The listing builds one solid part. Answer for the finished solid, in the listing's coordinates (mm). Face numbers are marked on the shaded views. A direction names the side the tool comes from. Round coordinates to 2 decimals unless told otherwise and drop trailing zeros. Order: outer loops, then holes, each group sorted by start corner. A loop starts at its lowest first (then second) coordinate and runs counter-clockwise, first axis right, second up. Notation, with made-up numbers: M 28.5,65.5 L 34.5,65.5 A22 ccw 34.5,96.5 Z; hole C -35,4 d1. An arc over 180 degrees is marked long. Write item = value, one per line. Start each with the question number.
(1) Straight lines are drawn through the part: probe 1 along Z at (x, y) = (-19.5, 24) (3 decimals); probe 2 along Z at (x, y) = (-16, 68); probe 3 along Z at (x, y) = (73.5, 7). For each, find the intervals that lie inside material, in ascending order. Write a range as from..to.
(2) A cutting plane is placed at A-A, the plane z = 56. Determine the outline of the cut face in (x, y).
(3) A cutting plane is placed at D-D, the plane x = 10. Determine the outline of the cut face in (y, z), and give its area (3 significant figures).
(4) For a pull along Y with two mould halves and no side action, classify the marked faces 6, 7, 8 and 9 as released by +Y, released by -Y, zero draft, split by the parting line, or undercut.
(5) Each of these flat-tipped pins is pushed along its axis until it touches: pin 1 (1.5 mm diameter, centred on x = 67.5, z = 33, fed in from -Y); pin 2 (9 mm diameter, centred on x = -15, y = 4, fed in from +Z); pin 3 (4 mm diameter, centred on y = 12.5, z = 11.5, fed in from +X); pin 4 (5 mm diameter, centred on y = 40, z = 80, fed in from +X). Where does it stop, or does it pass through?
(6) Which of the six approach directions +Z, -Z, +X, -X, +Y, -Y give full straight-line access (tool end or side, diameter ignored) to the marked faces 1, 2, 3, 4 and 5?
(7) A cutting plane is placed at B-B, the plane y = 20. Determine the outline of the cut face in (x, z) (3 decimals).
(8) A cutting plane is placed at C-C, the plane z = 83.5. Determine the outline of the cut face in (x, y).
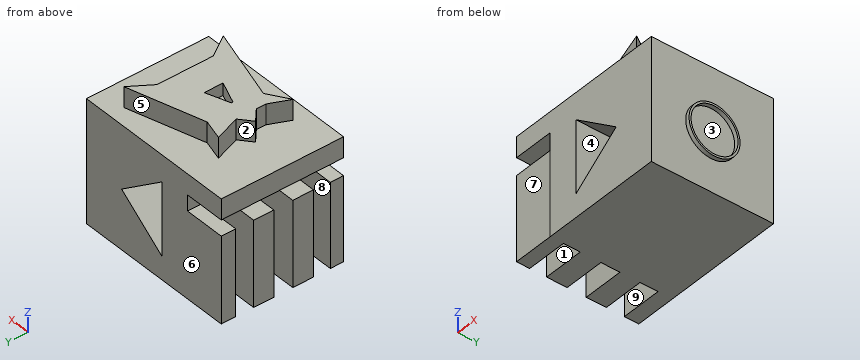
from build123d import *

# Parameters (mm, degrees)
F0_W      = 76.2
F0_H      = 76.2
F1_DEPTH  = 76.2
F2_W      = 12.539256
F2_H      = 53.205002
F2_W_2    = 12.878159
F2_W_3    = 8.237785
F2_H_2    = 52.527204
F2_W_4    = 8.993818
F2_H_3    = 53.543892
F2_W_5    = 76.2
F2_H_4    = 12.828036
F3_DEPTH  = 25.4
F5_DEPTH  = 254
F7_DEPTH  = 12.7
F9_DEPTH  = 7.62
F10_R     = 15.886225
F10_R_2   = 14.655787
F11_DEPTH = 2.54


with BuildPart() as f1:
    # F0 (on Top) → F1 (new body)
    with BuildSketch(Plane.XY):
        with Locations((38.1, 38.1)):
            Rectangle(F0_W, F0_H)
    extrude(amount=F1_DEPTH)

    # F2 (on face) → F3 (join)
    with BuildSketch(Plane(origin=(0, 0, 0), x_dir=(0, -1, 0), z_dir=(-1, 0, 0))):
        with Locations((-49.752893, 26.602501)):
            Rectangle(F2_W, F2_H)
        with Locations((-25.182727, 26.602501)):
            Rectangle(F2_W_2, F2_H)
        with Locations((-4.118892, 26.263602)):
            Rectangle(F2_W_3, F2_H_2)
        with Locations((-71.703091, 26.771946)):
            Rectangle(F2_W_4, F2_H_3)
        with Locations((-38.1, 69.785982)):
            Rectangle(F2_W_5, F2_H_4)
    extrude(amount=F3_DEPTH)

    # F4 (on face) → F5 (cut)
    with BuildSketch(Plane.XZ):
        Polygon((49.715646, 37.017897), (19.429348, 59.589423), (19.429348, 14.446371), align=None)
    extrude(amount=-F5_DEPTH, mode=Mode.SUBTRACT)

    # F6 (on face) → F7 (join)
    with BuildSketch(Plane.XY.offset(76.2)):
        Polygon((59.441991, 4.737339), (50.535221, 18.474905), (50.535221, 53.498153), (59.441991, 66.782832), (12.64369, 53.498153), (12.64369, 48.818324), (5.548463, 48.818324), (5.548463, 41.278802), (5.548463, 28.747914), (5.548463, 22.852812), (12.64369, 22.852812), (12.64369, 18.474905), align=None)
        Polygon((0, 10.469685), (12.64369, 18.474905), (12.64369, 22.852812), (5.548463, 22.852812), align=None)
        Polygon((12.64369, 48.818324), (12.64369, 53.498153), (0, 56.967318), (5.548463, 41.278802), (5.548463, 48.818324), align=None)
        Polygon((5.548463, 28.747914), (5.548463, 41.278802), (-1.681807, 35.226036), align=None)
    extrude(amount=F7_DEPTH)

    # F8 (on face) → F9 (cut)
    with BuildSketch(Plane.XY.offset(88.9)):
        Polygon((16.839748, 35.066836), (16.839748, 34.013547), (31.31187, 28.2102), (31.218205, 39.986227), align=None)
    extrude(amount=-F9_DEPTH, mode=Mode.SUBTRACT)

    # F10 (on face) → F11 (join)
    with BuildSketch(Plane.YZ.offset(76.2)):
        with Locations((37.34519, 36.212973)):
            Circle(F10_R)
        with Locations((37.34519, 36.212973)):
            Circle(F10_R_2, mode=Mode.SUBTRACT)
    extrude(amount=F11_DEPTH)


solid = f1.part
Reported:
q1.probe_1 = 0..53.205, 63.372..76.2
q1.probe_2 = 0..53.54, 63.37..76.2
q1.probe_3 = 0..76.2
q2.outline = M 0,0 L 19.43,0 L 19.43,76.2 L 0,76.2 Z; M 24.25,0 L 76.2,0 L 76.2,76.2 L 24.25,76.2 Z
q3.outline = M 0,0 L 76.2,0 L 76.2,76.2 L 54.22,76.2 L 54.22,88.9 L 16.8,88.9 L 16.8,76.2 L 0,76.2 Z
q3.area = 6,280 mm²
q4.face_6 = released by +Y
q4.face_7 = released by -Y
q4.face_8 = undercut
q4.face_9 = undercut
q5.pin_1 = 0
q5.pin_2 = 76.2
q5.pin_3 = 76.2
q5.pin_4 = 50.54
q6.face_1 = -Z, -X
q6.face_2 = +Z, -X
q6.face_3 = +X
q6.face_4 = +Y, -Y
q6.face_5 = +Z, +Y
q7.outline = M -25.4,0 L 76.2,0 L 76.2,76.2 L 50.535,76.2 L 50.535,88.9 L 4.27,88.9 L 4.27,76.2 L -25.4,76.2 L -25.4,63.372 L 0,63.372 L 0,53.205 L -25.4,53.205 Z; hole M 19.429,14.446 L 49.716,37.018 L 19.429,59.589 Z
q8.outline = M -1.68,35.23 L 5.55,28.75 L 5.55,22.85 L 0,10.47 L 12.64,18.47 L 59.44,4.74 L 50.54,18.47 L 50.54,53.5 L 59.44,66.78 L 12.64,53.5 L 0,56.97 L 5.55,41.28 Z; hole M 16.84,34.01 L 31.31,28.21 L 31.22,39.99 L 16.84,35.07 Z
